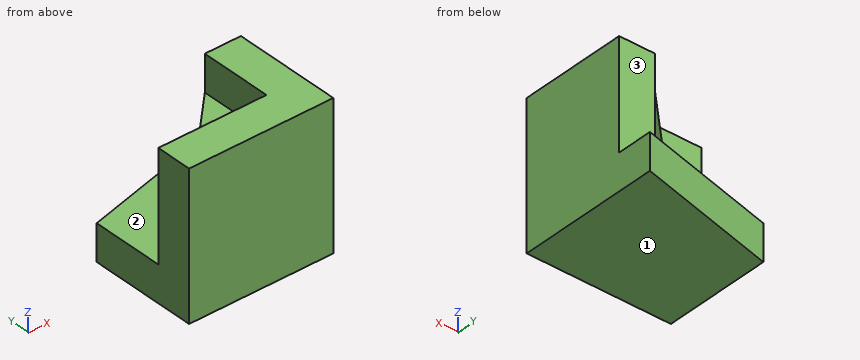
from build123d import *

# Parameters (mm, degrees)
SKETCH1_W           = 40
SKETCH1_H           = 40
BOSS_EXTRUDE1_DEPTH = 40
CUT_EXTRUDE1_DEPTH  = 40
SKETCH3_W           = 30
SKETCH3_H           = 10
CUT_EXTRUDE2_DEPTH  = 40
CUT_EXTRUDE6_DEPTH  = 30
SKETCH6_W           = 30
SKETCH6_H           = 20
CUT_EXTRUDE7_DEPTH  = 30
CUT_EXTRUDE9_DEPTH  = 10


with BuildPart() as part:
    # Sketch1 → Boss-Extrude1 (new body)
    with BuildSketch(Plane.XY):
        with Locations((20, 20)):
            Rectangle(SKETCH1_W, SKETCH1_H)
    extrude(amount=BOSS_EXTRUDE1_DEPTH)

    # Sketch2 → Cut-Extrude1 (cut)
    with BuildSketch(Plane.XY.offset(40)):
        Polygon((40, 40), (0, 30), (0, 40), align=None)
    extrude(amount=-CUT_EXTRUDE1_DEPTH, mode=Mode.SUBTRACT)

    # Sketch3 → Cut-Extrude2 (cut)
    with BuildSketch(Plane(origin=(40, 0, 0), x_dir=(0, 0, -1), z_dir=(1, 0, 0))):
        with Locations((-25, 35)):
            Rectangle(SKETCH3_W, SKETCH3_H)
    extrude(amount=-CUT_EXTRUDE2_DEPTH, mode=Mode.SUBTRACT)

    # Sketch4 → Cut-Extrude6 (cut)
    with BuildSketch(Plane.XY.offset(40)):
        Polygon((30, 30), (10, 30), (10, 10), align=None)
    extrude(amount=-CUT_EXTRUDE6_DEPTH, mode=Mode.SUBTRACT)

    # Sketch6 → Cut-Extrude7 (cut)
    with BuildSketch(Plane(origin=(10, 0, 0), x_dir=(0, 0, -1), z_dir=(1, 0, 0))):
        with Locations((-25, 20)):
            Rectangle(SKETCH6_W, SKETCH6_H)
    extrude(amount=-CUT_EXTRUDE7_DEPTH, mode=Mode.SUBTRACT)

    # Sketch7 → Cut-Extrude9 (cut)
    with BuildSketch(Plane.XY.offset(40)):
        Polygon((30, 30), (30, 10), (10, 10), align=None)
    extrude(amount=-CUT_EXTRUDE9_DEPTH, mode=Mode.SUBTRACT)


solid = part.part
Model file for the job. Use its own axes, mm. Face numbers are marked on the shaded views. A direction names the side the tool comes from. Give positions to 0.01 mm unless a question says otherwise; leave off trailing zeros. Loops run counter-clockwise (first coordinate to the right, second up) from the corner with the lowest first, then second, coordinate; pieces in that order, holes last.
Item 1: Drop flat-ended pins along their axis: P1, Ø12, axis at y = 35, z = 28, coming from the -X side; P2, Ø16, axis at x = 24, y = 18.5, coming from the +Z side; P3, Ø5, axis at x = 20, z = 24, coming from the +Y side; P4, Ø3, axis at x = 20.5, y = 26.5, coming from the +Z side. Give the stop position or say it passes through.
Check values:
P1: stops at x = 29
P2: stops at z = 40
P3: stops at y = 22.5
P4: stops at z = 10
Item 2: Which spindle directions (+Z, -Z, +X, -X, +Y, -Y) get a long thin tool onto all of the face, cutting with end or side? Do the marked faces 1, 2 and 3. Say none if no direction does.
Check values:
face 1: -Z, +X, -X, +Y, -Y
face 2: +Z, -X, +Y
face 3: +Z, +X, -X, +Y
Item 3: Slice it at A-A (y = 21.5). Write the cut outline in (x, z).
Check values:
outline: (0, 0) - (40, 0) - (40, 40) - (30, 40) - (30, 30) - (21.5, 30) - (21.5, 10) - (0, 10) - close
Item 4: Slice it at D-D (x = 9). Write the cut outline in (y, z).
Check values:
outline: (0, 0) - (32.25, 0) - (32.25, 10) - (10, 10) - (10, 40) - (0, 40) - close
Item 5: Slice it at C-C (z = 34). Write the cut outline in (x, y), plus the area to 3 significant figures.
Check values:
outline: (0, 0) - (40, 0) - (40, 30) - (30, 30) - (30, 10) - (0, 10) - close
area: 600 mm2
Item 6: Drill centre lines: line 1 along Y through (x, z) = (34.5, 34.5); line 2 along X through (y, z) = (27, 38); line 3 along Z through (x, y) = (38, 37). Where is each one in solid material? Low to high.
Check values:
line 1: y = 0 to 30
line 2: x = 30 to 40
line 3: z = 0 to 10
Item 7: Slice it at B-B (x = 16). Write the cut outline in (y, z), plus the area to 3 significant figures.
Check values:
outline: (0, 0) - (34, 0) - (34, 10) - (16, 10) - (16, 30) - (10, 30) - (10, 40) - (0, 40) - close
area: 760 mm2
